The model under review builds one solid part; all positions refer to its coordinate system, in mm. Round coordinates to 2 decimals unless told otherwise and drop trailing zeros. Write each loop counter-clockwise with the first axis right and the second up, starting at its lowest first coordinate (ties: lowest second). Pieces come first, ordered by that corner, then holes. Notation, with made-up numbers: M 30.25,-19.5 L 42.25,-19.5 A28 ccw 42.25,16.5 Z; hole C -19.5,8 d10. An arc over 180 degrees is marked long. One line per item, written item: value. Start each with the question number.
1) For P1, Ø0.6, axis at x = 63.5, y = 0.5, coming from the +Z side; P2, Ø1, axis at x = -57, y = 1.5, coming from the -Z side; P3, Ø0.6, axis at y = 0.5, z = 13.5, coming from the -X side, all flat-tipped, find the tip position at first contact; note any pin that passes through.
2) Take a section at B-B, the plane x = -2.5. Write out the cut boundary in (y, z), and give its area (3 significant figures).
3) Take a section at A-A, the plane z = 3.5. Write out the cut boundary in (x, y).
4) Wall thickness on probe 1 along X at (y, z) = (0.9, 3.5); probe 2 along Z at (x, y) = (56, 1.6); probe 3 along X at (y, z) = (1.9, -19): over which ranges is each line inside the solid? List them lowest first.
5) Take a section at C-C, the plane z = 18. Write out the cut boundary in (x, y).
from build123d import *

# Parameters (mm, degrees)
BOSS_EXTRUDE1_DEPTH = 2.1
SKETCH3_R           = 5.75
CUT_EXTRUDE1_DEPTH  = 75.87763351
SKETCH4_W           = 1.5
SKETCH4_H           = 12
SKETCH4_W_2         = 30
SKETCH4_H_2         = 1.5
CUT_EXTRUDE2_DEPTH  = 75.87763351


with BuildPart() as part:
    # Sketch1 → Boss-Extrude1 (new body)
    with BuildSketch(Plane(origin=(0, 0, 0), x_dir=(1, 0, 0), z_dir=(0, 1, 0))):
        Polygon((-70, 23.5), (-49, 23.5), (-49, 26.5), (-21, 26.5), (-21, 23.5), (21, 23.5), (21, 26.5), (49, 26.5), (49, 23.5), (70, 23.5), (70, -23.5), (-70, -23.5), align=None)
    extrude(amount=BOSS_EXTRUDE1_DEPTH)

    # Sketch3 → Cut-Extrude1 (cut, through all)
    with BuildSketch(Plane(origin=(0, 2.1, 0), x_dir=(1, 0, 0), z_dir=(0, 1, 0))):
        with Locations(Location((-40, -3.5, 0), (0, 0, 270))):
            Circle(SKETCH3_R)
    extrude(amount=-CUT_EXTRUDE1_DEPTH, mode=Mode.SUBTRACT)

    # Sketch4 → Cut-Extrude2 (cut, through all)
    with BuildSketch(Plane(origin=(0, 2.1, 0), x_dir=(1, 0, 0), z_dir=(0, 1, 0))):
        with Locations((-69.25, 17.5)):
            Rectangle(SKETCH4_W, SKETCH4_H)
        Polygon((-70, -5.5), (-70, -23.5), (-60, -23.5), (-60, -22), (-68.5, -22), (-68.5, -5.5), align=None)
        with Locations((-25, -22.75)):
            Rectangle(SKETCH4_W_2, SKETCH4_H_2)
        with Locations((25, -22.75)):
            Rectangle(SKETCH4_W_2, SKETCH4_H_2)
        Polygon((60, -23.5), (70, -23.5), (70, -5.5), (68.5, -5.5), (68.5, -22), (60, -22), align=None)
        with Locations((69.25, 17.5)):
            Rectangle(SKETCH4_W, SKETCH4_H)
    extrude(amount=-CUT_EXTRUDE2_DEPTH, mode=Mode.SUBTRACT)


solid = part.part
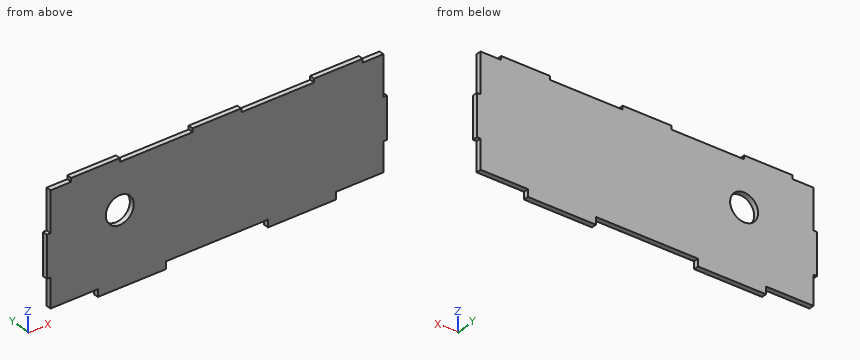
Checked values:
1. P1: stops at z = 22
1. P2: stops at z = -23.5
1. P3: stops at x = -68.5
2. outline: M 0,-23.5 L 2.1,-23.5 L 2.1,23.5 L 0,23.5 Z
2. area: 98.7 mm2
3. outline: M -70,0 L -45.75,0 L -45.75,2.1 L -70,2.1 Z; M -34.25,0 L 70,0 L 70,2.1 L -34.25,2.1 Z
4. probe 1: x = -70 to -45.75, -34.25 to 70
4. probe 2: z = -23.5 to 23.5
4. probe 3: x = -68.5 to 68.5
5. outline: M -68.5,0 L 68.5,0 L 68.5,2.1 L -68.5,2.1 Z
